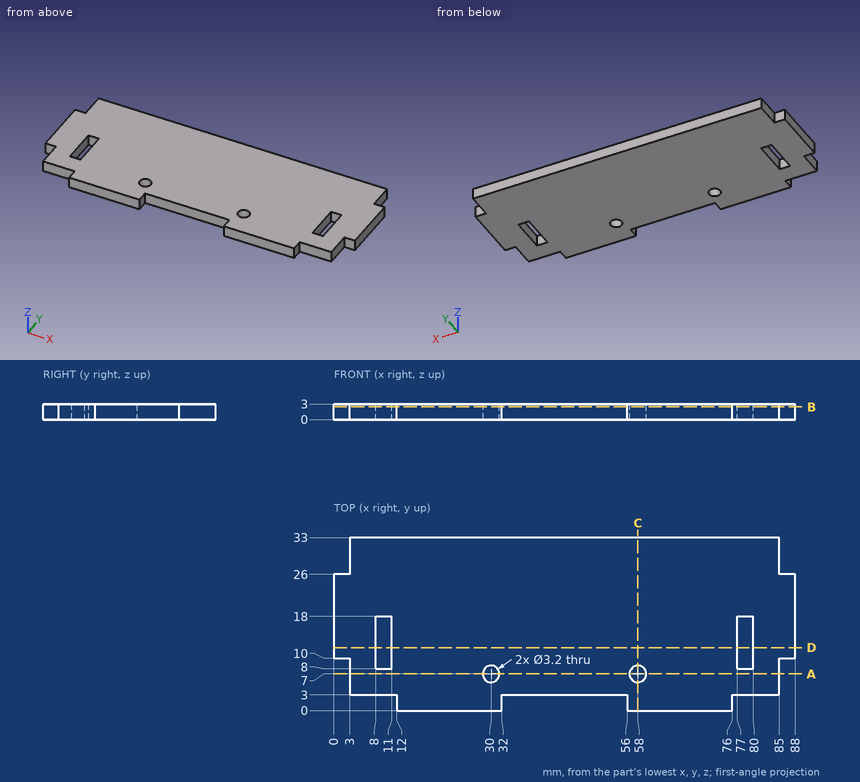
Job drawing, mm, ordinate dimensions from the low corner. One solid piece. Coordinates: 2 decimals unless noted, no trailing zeros. Write each loop counter-clockwise with the first axis right and the second up, starting at its lowest first coordinate (ties: lowest second). Pieces come first, ordered by that corner, then holes. Notation, with made-up numbers: M 70.5,8.25 L 78.5,8.25 A9 cw 78.5,21.25 Z; hole C 1.25,-34.5 d11. An arc over 180 degrees is marked long. Answer as a JSON object with one key per item and string values. Group by question number.
1) Saw through at A-A (y = 7). Write the cut outline in (x, z), plus the area to 3 significant figures.
2) Saw through at D-D (y = 12). Write the cut outline in (x, z), plus the area to 3 significant figures.
3) Saw through at B-B (z = 2.45). Give the number of separate pieces and of enclosed holes in the cut face, plus the area to 3 significant figures.
4) Pin check, flat tips, straight feed: pin 1 Ø1.5 at (x, z) = (87, 2) entering from +Y; pin 2 Ø0.9 at (x, z) = (9, 1) entering from -Y; pin 3 Ø0.9 at (y, z) = (1.5, 1) entering from +X. Stop position of each tip, or through.
5) Saw through at C-C (x = 58). Write the cut outline in (y, z), plus the area to 3 significant figures.
6) Wall check: line 1 (X direction, y = 12.5, z = 0.2); line 2 (Y direction, x = 79, z = 1.5); line 3 (Y direction, x = 58, z = 1.4). Give the ranges that are in metal, low to high. Write a range as from..to.
Values follow:
{
 "1": {"outline": "M 3,0 L 28.4,0 L 28.4,3 L 3,3 Z; M 31.6,0 L 56.4,0 L 56.4,3 L 31.6,3 Z; M 59.6,0 L 85,0 L 85,3 L 59.6,3 Z", "area": "227 mm2"},
 "2": {"outline": "M 0,0 L 8,0 L 8,3 L 0,3 Z; M 11,0 L 77,0 L 77,3 L 11,3 Z; M 80,0 L 88,0 L 88,3 L 80,3 Z", "area": "246 mm2"},
 "3": {"separate pieces": "1", "enclosed holes": "4", "area": "2,600 mm2"},
 "4": {"pin 1": "stops at y = 26", "pin 2": "stops at y = 3", "pin 3": "stops at x = 76"},
 "5": {"outline": "M 0,0 L 5.4,0 L 5.4,3 L 0,3 Z; M 8.6,0 L 33,0 L 33,3 L 8.6,3 Z", "area": "89.4 mm2"},
 "6": {"line 1": "x = 0..8, 11..77, 80..88", "line 2": "y = 3..8, 18..33", "line 3": "y = 0..5.4, 8.6..33"}
}
